from build123d import *

# Parameters (mm, degrees)
BOSS_EXTRUDE1_DEPTH      = 101.6
BOSS_EXTRUDE1_DEPTH_BACK = 101.6
SKETCH1_W                = 38.1
SKETCH1_H                = 38.1
SKETCH2_W                = 38.1
SKETCH2_H                = 38.1
BOSS_EXTRUDE2_DEPTH      = 327.66000001


with BuildPart() as part:
    # Sketch1 → Boss-Extrude1 (new, two sides: drawn at the far end of the back side and taken through both)
    with BuildSketch(Plane.XY.offset(-BOSS_EXTRUDE1_DEPTH_BACK)):
        with Locations((-19.05, -19.05)):
            Rectangle(SKETCH1_W, SKETCH1_H)
    extrude(amount=BOSS_EXTRUDE1_DEPTH + BOSS_EXTRUDE1_DEPTH_BACK)

    # Sketch2 → Boss-Extrude2 (add)
    with BuildSketch(Plane.ZY.offset(38.1)):
        with Locations((-82.55, -19.05)):
            Rectangle(SKETCH2_W, SKETCH2_H)
        with Locations((82.55, -19.05)):
            Rectangle(SKETCH2_W, SKETCH2_H)
    extrude(amount=BOSS_EXTRUDE2_DEPTH)


solid = part.part
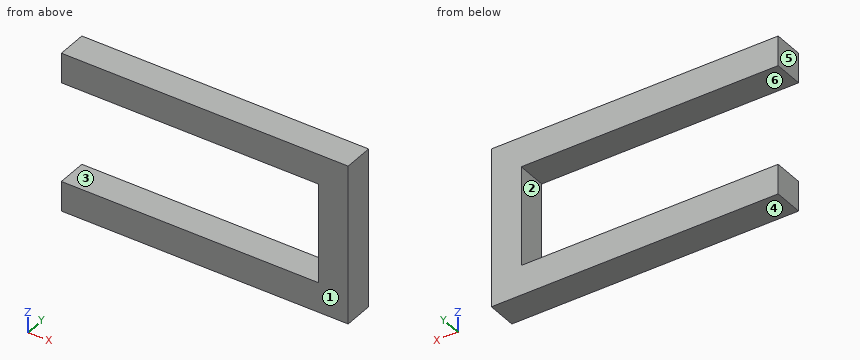
Check sheet for the modelled part. Datum: model origin and axes. Units: mm. Face numbers are marked on the shaded views. A direction names the side the tool comes from. Coordinates: 2 decimals unless noted, no trailing zeros. Loops run counter-clockwise (first coordinate to the right, second up) from the corner with the lowest first, then second, coordinate; pieces in that order, holes last. Notation, with made-up numbers: (25, 51) -> (74, 51) arc R29 cw to (74, 87) -> close; hole circle Ø2 at (-15.75, 73.5). An arc over 180 degrees is marked (long way). Write item = value, one per line. Start each with the question number.
1. Depth check by flat-ended pin: P1, Ø3, axis at y = -10.5, z = -50.5, coming from the -X side. Enter the tip coordinate at first touch or a pass-through.
2. Tool access check on the marked faces 5 and 6. Record the directions out of +Z, -Z, +X, -X, +Y, -Y that give a thin tool (end or side, any length) a straight path to the whole face; none if there is none.
3. Draft check along Z on the marked faces 1, 2, 3 and 4. Enter one of: released by +Z, released by -Z, zero draft, split by the parting line, or undercut.
4. Material ranges on line 1 (Z direction, x = -228, y = -33); line 2 (X direction, y = -7, z = -27), recorded low to high.
5. Section check A-A on x = -152.5. Record the cut outline in (y, z).
6. Section check B-B on y = -26.5. Record the cut outline in (x, z), then the cut area to 3 significant figures.
7. Section check C-C on z = -29. Record the cut outline in (x, y), then the cut area to 3 significant figures.
Responses:
q1.P1 = -38.1
q2.face_5 = +Z, -Z, -X, +Y, -Y
q2.face_6 = -X, +Y, -Y
q3.face_1 = zero draft
q3.face_2 = undercut
q3.face_3 = undercut
q3.face_4 = released by -Z
q4.line_1 = -101.6 to -63.5, 63.5 to 101.6
q4.line_2 = -38.1 to 0
q5.outline = (-38.1, -101.6) -> (0, -101.6) -> (0, -63.5) -> (-38.1, -63.5) -> close; (-38.1, 63.5) -> (0, 63.5) -> (0, 101.6) -> (-38.1, 101.6) -> close
q6.outline = (-365.76, -101.6) -> (0, -101.6) -> (0, 101.6) -> (-365.76, 101.6) -> (-365.76, 63.5) -> (-38.1, 63.5) -> (-38.1, -63.5) -> (-365.76, -63.5) -> close
q6.area = 32,700 mm2
q7.outline = (-38.1, -38.1) -> (0, -38.1) -> (0, 0) -> (-38.1, 0) -> close
q7.area = 1,450 mm2
